Geometry: final body of the model. Coordinates: model frame, mm. A direction names the side the tool comes from. Coordinates: 2 decimals unless noted, no trailing zeros. Write each loop counter-clockwise with the first axis right and the second up, starting at its lowest first coordinate (ties: lowest second). Pieces come first, ordered by that corner, then holes. Notation, with made-up numbers: (66, -32) -> (70, -32) arc R26 ccw to (70, -13) -> close; hole circle Ø2 at (38, -11.5). An arc over 180 degrees is marked (long way). One line per item, written item: value.
```python
from build123d import *

# Parameters (mm, degrees)
BOSS_EXTRUDE2_DEPTH  = 4
SKETCH2_W            = 390
SKETCH2_H            = 480
BOSS_EXTRUDE3_DEPTH  = 4
SKETCH3_W            = 380
SKETCH3_H            = 470
BOSS_EXTRUDE4_DEPTH  = 4
SKETCH4_W            = 370
SKETCH4_H            = 460
BOSS_EXTRUDE5_DEPTH  = 4
SKETCH5_W            = 360
SKETCH5_H            = 450
BOSS_EXTRUDE6_DEPTH  = 4
SKETCH6_W            = 280
SKETCH6_H            = 370
CUT_EXTRUDE1_DEPTH   = 4
SKETCH7_W            = 270
SKETCH7_H            = 360
CUT_EXTRUDE2_DEPTH   = 4
SKETCH8_W            = 260
SKETCH8_H            = 350
CUT_EXTRUDE3_DEPTH   = 4
SKETCH9_W            = 250
SKETCH9_H            = 340
CUT_EXTRUDE4_DEPTH   = 4
SKETCH11_W           = 190
SKETCH11_H           = 280
BOSS_EXTRUDE7_DEPTH  = 4
SKETCH12_W           = 180
SKETCH12_H           = 270
BOSS_EXTRUDE8_DEPTH  = 4
SKETCH13_W           = 170
SKETCH13_H           = 260
BOSS_EXTRUDE9_DEPTH  = 4
SKETCH14_W           = 160
SKETCH14_H           = 250
BOSS_EXTRUDE10_DEPTH = 4
SKETCH15_W           = 20
SKETCH15_H           = 20
BOSS_EXTRUDE11_DEPTH = 5
SKETCH16_W           = 15
SKETCH16_H           = 15
BOSS_EXTRUDE12_DEPTH = 5
SKETCH17_W           = 10
SKETCH17_H           = 10
BOSS_EXTRUDE13_DEPTH = 20
BOSS_EXTRUDE14_REACH = 302
SKETCH18_W           = 10
SKETCH18_H           = 10
CUT_EXTRUDE6_DEPTH   = 3


with BuildPart() as part:
    # Sketch1 → Boss-Extrude2 (new body)
    with BuildSketch(Plane.XY):
        Polygon((200, 0), (200, -20), (200, -245), (-200, -245), (-200, -20), (-200, 0), (-200, 245), (200, 245), align=None)
    extrude(amount=BOSS_EXTRUDE2_DEPTH)

    # Sketch2 → Boss-Extrude3 (add)
    with BuildSketch(Plane.XY.offset(4)):
        Rectangle(SKETCH2_W, SKETCH2_H)
    extrude(amount=BOSS_EXTRUDE3_DEPTH)

    # Sketch3 → Boss-Extrude4 (add)
    with BuildSketch(Plane.XY.offset(8)):
        Rectangle(SKETCH3_W, SKETCH3_H)
    extrude(amount=BOSS_EXTRUDE4_DEPTH)

    # Sketch4 → Boss-Extrude5 (add)
    with BuildSketch(Plane.XY.offset(12)):
        Rectangle(SKETCH4_W, SKETCH4_H)
    extrude(amount=BOSS_EXTRUDE5_DEPTH)

    # Sketch5 → Boss-Extrude6 (add)
    with BuildSketch(Plane.XY.offset(16)):
        Rectangle(SKETCH5_W, SKETCH5_H)
    extrude(amount=BOSS_EXTRUDE6_DEPTH)

    # Sketch6 → Cut-Extrude1 (cut)
    with BuildSketch(Plane.XY.offset(20)):
        Rectangle(SKETCH6_W, SKETCH6_H)
    extrude(amount=-CUT_EXTRUDE1_DEPTH, mode=Mode.SUBTRACT)

    # Sketch7 → Cut-Extrude2 (cut)
    with BuildSketch(Plane.XY.offset(16)):
        Rectangle(SKETCH7_W, SKETCH7_H)
    extrude(amount=-CUT_EXTRUDE2_DEPTH, mode=Mode.SUBTRACT)

    # Sketch8 → Cut-Extrude3 (cut)
    with BuildSketch(Plane.XY.offset(12)):
        Rectangle(SKETCH8_W, SKETCH8_H)
    extrude(amount=-CUT_EXTRUDE3_DEPTH, mode=Mode.SUBTRACT)

    # Sketch9 → Cut-Extrude4 (cut)
    with BuildSketch(Plane.XY.offset(8)):
        Rectangle(SKETCH9_W, SKETCH9_H)
    extrude(amount=-CUT_EXTRUDE4_DEPTH, mode=Mode.SUBTRACT)

    # Sketch11 → Boss-Extrude7 (add)
    with BuildSketch(Plane.XY.offset(4)):
        Rectangle(SKETCH11_W, SKETCH11_H)
    extrude(amount=BOSS_EXTRUDE7_DEPTH)

    # Sketch12 → Boss-Extrude8 (add)
    with BuildSketch(Plane.XY.offset(8)):
        Rectangle(SKETCH12_W, SKETCH12_H)
    extrude(amount=BOSS_EXTRUDE8_DEPTH)

    # Sketch13 → Boss-Extrude9 (add)
    with BuildSketch(Plane.XY.offset(12)):
        Rectangle(SKETCH13_W, SKETCH13_H)
    extrude(amount=BOSS_EXTRUDE9_DEPTH)

    # Sketch14 → Boss-Extrude10 (add)
    with BuildSketch(Plane.XY.offset(16)):
        Rectangle(SKETCH14_W, SKETCH14_H)
    extrude(amount=BOSS_EXTRUDE10_DEPTH)

    # Sketch15 → Boss-Extrude11 (add)
    with BuildSketch(Plane.XY.offset(20)):
        with Locations((160, 60)):
            Rectangle(SKETCH15_W, SKETCH15_H)
        with Locations((160, -60)):
            Rectangle(SKETCH15_W, SKETCH15_H)
    extrude(amount=BOSS_EXTRUDE11_DEPTH)

    # Sketch16 → Boss-Extrude12 (add)
    with BuildSketch(Plane.XY.offset(25)):
        with Locations((160, 60)):
            Rectangle(SKETCH16_W, SKETCH16_H)
        with Locations((160, -60)):
            Rectangle(SKETCH16_W, SKETCH16_H)
    extrude(amount=BOSS_EXTRUDE12_DEPTH)

    # Sketch17 → Boss-Extrude13 (add)
    with BuildSketch(Plane.XY.offset(30)):
        with Locations((160, 60)):
            Rectangle(SKETCH17_W, SKETCH17_H)
        with Locations((160, -60)):
            Rectangle(SKETCH17_W, SKETCH17_H)
    extrude(amount=BOSS_EXTRUDE13_DEPTH)

    # Sketch18 → Boss-Extrude14 (add, up to next)
    with BuildSketch(Plane.XZ.offset(-55), mode=Mode.PRIVATE) as boss_extrude14_sk1:
        with Locations((160, 45)):
            Rectangle(SKETCH18_W, SKETCH18_H)
    boss_extrude14_tool1 = extrude(boss_extrude14_sk1.sketch, amount=BOSS_EXTRUDE14_REACH, mode=Mode.PRIVATE) - part.part
    add(boss_extrude14_tool1.solids().sort_by_distance((160, 55, 45))[0])

    # Sketch19 → Cut-Extrude6 (cut)
    with BuildSketch(Plane(origin=(0, 0, 0), x_dir=(-1, 0, 0), z_dir=(0, 0, -1))):
        with BuildLine():
            Line((165, 191.875), (165, 101.875))
            ThreePointArc((165, 101.875), (180, 91.875), (195, 101.875))
            Line((195, 101.875), (195, 141.875))
            Line((195, 141.875), (200, 141.875))
            Line((200, 141.875), (200, 191.875))
            Line((200, 191.875), (165, 191.875))
        make_face()
        with BuildLine():
            Line((165, -108.125), (165, -198.125))
            ThreePointArc((165, -198.125), (180, -208.125), (195, -198.125))
            Line((195, -198.125), (195, -158.125))
            Line((195, -158.125), (200, -158.125))
            Line((200, -158.125), (200, -108.125))
            Line((200, -108.125), (165, -108.125))
        make_face()
    extrude(amount=-CUT_EXTRUDE6_DEPTH, mode=Mode.SUBTRACT)


solid = part.part
```
(1) Line query: line 1 (Y direction, x = -50, z = 11); line 2 (X direction, y = 6, z = 4.5); line 3 (X direction, y = -144.5, z = 10). Output: solid intervals per line, ascending. Write a range as [from, to].
Responses:
line 1: y = [-235, -175], [-135, 135], [175, 235]
line 2: x = [-195, -125], [-95, 95], [125, 195]
line 3: x = [-190, -130], [130, 190]
(2) First-contact query: pin 1 (1.5 mm diameter, centred on x = 162.5, z = 27, fed in from +Y); pin 2 (1.5 mm diameter, centred on y = 64.5, z = 23, fed in from +X); pin 3 (3 mm diameter, centred on x = 143.5, y = -132, fed in from +Z). Flat tips, straight axial feed; report the tip coordinate or a pass-through.
Responses:
pin 1: stops at y = 67.5
pin 2: stops at x = 170
pin 3: stops at z = 20
(3) Reachability of faces 5 (the flat face through (-131, 1, 12)), 6 (the flat face through (155, 1, 44)), 7 (the flat face through (165, 1, 44)), 8 (the flat face through (160, 1, 50)) from +Z, -Z, +X, -X, +Y, -Y: full face, straight path, thin tool, end or side. Return the list, or none.
Responses:
face 5: +Z
face 6: +Z, -X, +Y, -Y
face 7: +Z, +X, +Y, -Y
face 8: +Z, +X, -X, +Y, -Y
(4) Pull-direction query (Z, two-part tool) for faces 1 (the flat face through (-135.5, 0.9, 16)), 2 (the flat face through (169, 60, 25)), 3 (the flat face through (160, -55, 35)), 4 (the flat face through (3, 3, 0)); classes: released by +Z, released by -Z, zero draft, split by the parting line, or undercut.
Responses:
face 1: released by +Z
face 2: undercut
face 3: undercut
face 4: released by -Z
(5) Section A-A (y = 215). Return the cut outline in (x, z).
Responses:
outline: (-200, 0) -> (200, 0) -> (200, 4) -> (195, 4) -> (195, 8) -> (190, 8) -> (190, 12) -> (185, 12) -> (185, 16) -> (180, 16) -> (180, 20) -> (-180, 20) -> (-180, 16) -> (-185, 16) -> (-185, 12) -> (-190, 12) -> (-190, 8) -> (-195, 8) -> (-195, 4) -> (-200, 4) -> close
